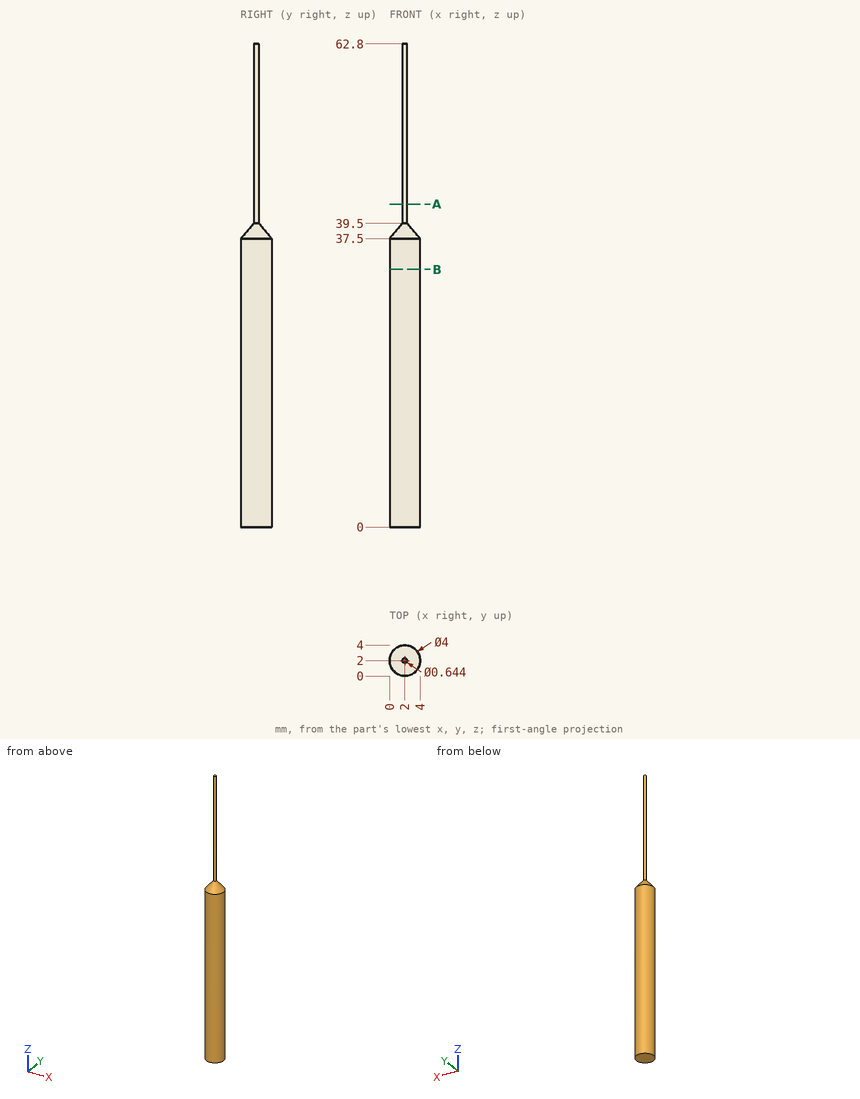
Design review of the part shown in the three views and the two pictorial views. Dimensions are in mm from the part's minimum x, y and z. Give positions to 0.01 mm unless a question says otherwise; leave off trailing zeros. Write each loop counter-clockwise with the first axis right and the second up, starting at its lowest first coordinate (ties: lowest second). Pieces come first, ordered by that corner, then holes.
Item 1: Insertion check: P1, Ø1, axis at y = 1, z = 16.5, coming from the +X side. The pin has a flat end and moves straight along its axis. Give the tip position at first contact, or say it passes through.
Item 2: Wall thickness on probe 1 along Y at (x, z) = (2, 50.5); probe 2 along X at (y, z) = (2.1, 28); probe 3 along Y at (x, z) = (1.45, 24): over which ranges is each line inside the solid? List them lowest first.
Item 3: Take a section at A-A (z = 42). Give the boundary of the cut face in (x, y).
Item 4: Take a section at B-B (z = 33.5). Give the boundary of the cut face in (x, y).
Established:
1. P1: stops at x = 3.94
2. probe 1: y = 1.68 to 2.32
2. probe 2: x = 0 to 4
2. probe 3: y = 0.08 to 3.92
3. outline: circle Ø0.64 at (2, 2)
4. outline: circle Ø4 at (2, 2)
